```python
from build123d import *
from OCP.BRepFilletAPI import BRepFilletAPI_MakeChamfer

# Parameters (mm, degrees)
SKETCH1_W           = 84
SKETCH1_H           = 66
BOSS_EXTRUDE1_DEPTH = 3
CHAMFER2_SIZE       = 6
CHAMFER4_SIZE       = 3
CHAMFER4_SIZE_2     = 6
SKETCH2_R           = 1.75
CUT_EXTRUDE1_DEPTH  = 54.4976635
SKETCH3_W           = 69
SKETCH3_H           = 44
CUT_EXTRUDE2_DEPTH  = 10


with BuildPart() as part:
    # Sketch1 → Boss-Extrude1 (new body)
    with BuildSketch(Plane.XY):
        Rectangle(SKETCH1_W, SKETCH1_H)
    extrude(amount=BOSS_EXTRUDE1_DEPTH)

    # Chamfer2
    chamfer2_edges = [part.edges().sort_by_distance(p)[0] for p in [
        (42, -33, 1.5),
        (-42, -33, 1.5),
        (-42, 33, 1.5),
        (42, 33, 1.5),
    ]]
    chamfer(chamfer2_edges, length=CHAMFER2_SIZE)

    # Chamfer4
    chamfer4_edges_1 = [part.edges().sort_by_distance(p)[0] for p in [
        (0, -33, 3),
    ]]
    chamfer4_side_1 = [part.faces().sort_by_distance(p)[0] for p in [
        (0, -33, 2.94),
    ]]
    chamfer4_edges_2 = [part.edges().sort_by_distance(p)[0] for p in [
        (0, 33, 3),
    ]]
    chamfer4_side_2 = [part.faces().sort_by_distance(p)[0] for p in [
        (0, 32.94, 3),
    ]]
    chamfer4 = BRepFilletAPI_MakeChamfer(part.part.solid().wrapped)
    for e in chamfer4_edges_1:
        chamfer4.Add(CHAMFER4_SIZE - 0.0001, CHAMFER4_SIZE_2 - 0.0001, e.wrapped, chamfer4_side_1[0].wrapped)
    for e in chamfer4_edges_2:
        chamfer4.Add(CHAMFER4_SIZE_2 - 0.0001, CHAMFER4_SIZE - 0.0001, e.wrapped, chamfer4_side_2[0].wrapped)
    add(Compound.cast(chamfer4.Shape()), mode=Mode.REPLACE)  # a hair under: the kernel refuses the full size

    # Sketch2 → Cut-Extrude1 (cut, through all)
    with BuildSketch(Plane.XY.offset(3)):
        with Locations((-39, -19)):
            Circle(SKETCH2_R)
        with Locations(Location((39, -19, 0), (0, 0, 180))):
            Circle(SKETCH2_R)
        with Locations((39, 16)):
            Circle(SKETCH2_R)
        with Locations(Location((-39, 16, 0), (0, 0, 180))):
            Circle(SKETCH2_R)
    extrude(amount=-CUT_EXTRUDE1_DEPTH, mode=Mode.SUBTRACT)

    # Sketch3 → Cut-Extrude2 (cut)
    with BuildSketch(Plane.XY.offset(3)):
        with Locations((-7.5, 11)):
            Rectangle(SKETCH3_W, SKETCH3_H)
    extrude(amount=-CUT_EXTRUDE2_DEPTH, mode=Mode.SUBTRACT)


solid = part.part
```
Geometry: final body of the model. Coordinates: model frame, mm. A direction names the side the tool comes from. Round coordinates to 2 decimals unless told otherwise and drop trailing zeros. Order: outer loops, then holes, each group sorted by start corner. A loop starts at its lowest first (then second) coordinate and runs counter-clockwise, first axis right, second up. Notation, with made-up numbers: M -26,33.5 L 13,33.5 A6 ccw 13,43.5 Z; hole C -27,-17.5 d4. An arc over 180 degrees is marked long. One line per item, written item: value.
(1) Cut plane B-B (x = 39). Return the cut outline in (y, z).
Result sheet:
outline: M -30,0 L -20.75,0 L -20.75,3 L -27,3 L -30,1.5 Z; M -17.25,0 L 14.25,0 L 14.25,3 L -17.25,3 Z; M 17.75,0 L 30,0 L 30,1.5 L 27,3 L 17.75,3 Z
(2) Cut plane A-A (y = 16). Return the cut outline in (x, z), and give its area (3 significant figures).
Result sheet:
outline: M 27,0 L 37.25,0 L 37.25,3 L 27,3 Z; M 40.75,0 L 42,0 L 42,3 L 40.75,3 Z
area: 34.5 mm2
(3) Cut plane C-C (y = -19). Return the cut outline in (x, z).
Result sheet:
outline: M -42,0 L -40.75,0 L -40.75,3 L -42,3 Z; M -37.25,0 L 37.25,0 L 37.25,3 L -37.25,3 Z; M 40.75,0 L 42,0 L 42,3 L 40.75,3 Z
(4) Cut plane D-D (z = 1.65). Return the cut outline in (x, y).
Result sheet:
outline: M -42,-27 L -39.3,-29.7 L 39.3,-29.7 L 42,-27 L 42,27 L 39.3,29.7 L 27,29.7 L 27,-11 L -42,-11 Z; hole C -39,-19 d3.5; hole C 39,-19 d3.5; hole C 39,16 d3.5
(5) Line query: probe 1 along Y at (x, z) = (39, 1.65); probe 2 along Y at (x, z) = (39, 1.2); probe 3 along X at (y, z) = (18, 1.35). Output: solid intervals per line, ascending. Write a range as [from, to].
Result sheet:
probe 1: [-29.7, -20.75], [-17.25, 14.25], [17.75, 29.7]
probe 2: [-30, -20.75], [-17.25, 14.25], [17.75, 30]
probe 3: [27, 42]
(6) Pull-direction query (X, two-part tool) for faces 3 (the cylindrical face through (-38.1, -17.5, 1.5)), 4 (the flat face through (-42, -19, 1)), 5 (the flat face through (9, -14, 0)); classes: pulls with the +X half, pulls with the -X half, needs draft (parallel to the pull), parting line crosses it, or undercut.
Result sheet:
face 3: undercut
face 4: pulls with the -X half
face 5: needs draft
(7) Pin query (flat end, axial travel): P1, Ø4, axis at x = 39, y = -19, coming from the -Z side; P2, Ø1, axis at x = 10, z = 0.5, coming from the +Y side; P3, Ø3, axis at x = 39, y = 16, coming from the +Z side. Return the tip coordinate at first contact, or that it passes through.
Result sheet:
P1: z = 0
P2: y = -11
P3: through
(8) Reachability of faces 1 (the flat face through (27, 11, 2)), 2 (the flat face through (42, 0, 1)) from +Z, -Z, +X, -X, +Y, -Y: full face, straight path, thin tool, end or side. Return the list, or none.
Result sheet:
face 1: +Z, -Z, -X, +Y
face 2: +Z, -Z, +X, +Y, -Y
